from build123d import *

# Parameters (mm, degrees)
ESQUISSE2_R             = 7
BOSS_EXTRU_2_DEPTH      = 22
ENL_V_MAT_EXTRU_1_DEPTH = 19
ESQUISSE5_R             = 5.5
ENL_V_MAT_EXTRU_2_DEPTH = 45
ENL_V_START             = -12
ENL_V_MAT_EXTRU_3_DEPTH = 24


with BuildPart() as part:
    # Esquisse2 → Boss.-Extru.2 (new body, symmetric)
    with BuildSketch(Plane.XY):
        with BuildLine():
            Line((51.296980053, -19), (57, -19))
            Line((57, -19), (86, 15))
            Line((86, 15), (86, 34))
            Line((86, 34), (81, 39))
            Line((81, 39), (57, 39))
            ThreePointArc((57, 39), (48.490791592, 29.99016727), (36.246410316, 28.077357637))
            Line((36.246410316, 28.077357637), (14, 32))
            Line((14, 32), (7, 32))
            Line((7, 32), (0, 25))
            Line((0, 25), (0, 7))
            Line((0, 7), (7, 0))
            Line((7, 0), (39.575538911, 0))
            ThreePointArc((39.575538911, 0), (42.840774692, -1.213413768), (44.521177653, -4.264705882))
            ThreePointArc((44.521177653, -4.264705882), (46.858007856, -12.115672061), (51.296980053, -19))
        make_face()
        with Locations((14, 14)):
            Circle(ESQUISSE2_R, mode=Mode.SUBTRACT)
    extrude(amount=BOSS_EXTRU_2_DEPTH, both=True)

    # Esquisse4 → Enlèv. mat.-Extru.1 (cut)
    with BuildSketch(Plane.XY.offset(22)):
        Polygon((34, 32), (0, 32), (0, -19), (86, -19), (86, 0), (34, 0), align=None)
    extrude(amount=-ENL_V_MAT_EXTRU_1_DEPTH, mode=Mode.SUBTRACT)

    # Esquisse5 → Enlèv. mat.-Extru.2 (cut, through all)
    with BuildSketch(Plane.XY.offset(22)):
        with Locations((72, 25)):
            Circle(ESQUISSE5_R)
    extrude(amount=-ENL_V_MAT_EXTRU_2_DEPTH, mode=Mode.SUBTRACT)

    # Esquisse14 → Enlèv. mat.-Extru.3 (cut)
    with BuildSketch(Plane(origin=(0, 0, -22), x_dir=(-1, 0, 0), z_dir=(0, 0, -1)).offset(ENL_V_START)):
        with BuildLine():
            Line((-75.764705882, 3), (-86, 15))
            Line((-86, 15), (-86, 34))
            Line((-86, 34), (-81, 39))
            Line((-81, 39), (-57, 39))
            ThreePointArc((-57, 39), (-53.002548038, 33.285750119), (-47.224051208, 29.381745985))
            ThreePointArc((-47.224051208, 29.381745985), (-58.169717695, 12.59414375), (-75.764705882, 3))
        make_face()
    extrude(amount=-ENL_V_MAT_EXTRU_3_DEPTH, mode=Mode.SUBTRACT)


solid = part.part
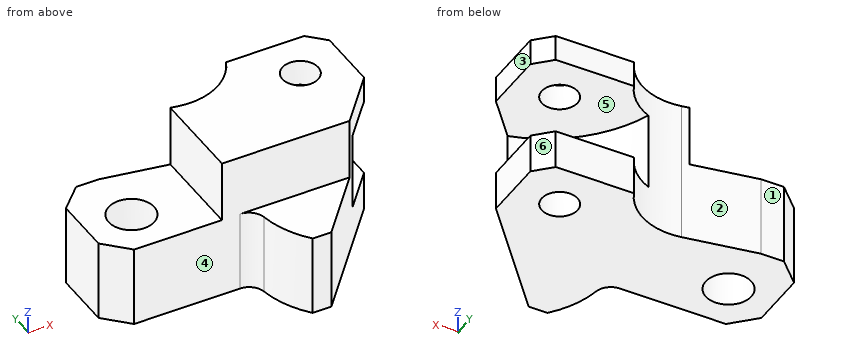
For this review, take the finished solid that the model builds, in its own axes (mm). Face numbers are marked on the shaded views. A direction names the side the tool comes from. Round coordinates to 2 decimals unless told otherwise and drop trailing zeros. Write each loop counter-clockwise with the first axis right and the second up, starting at its lowest first coordinate (ties: lowest second). Pieces come first, ordered by that corner, then holes. Notation, with made-up numbers: (67.25, -26.5) -> (75.25, -26.5) arc R11 cw to (75.25, -20.5) -> close; hole circle Ø8 at (25.5, 8). An arc over 180 degrees is marked (long way). Use CSV: the item, a comma, the result in double quotes.
(1) Consider section B-B, the plane y = 14. Give the boundary of the cut face in (x, z).
Computed values:
outline,"(0, -22) -> (7, -22) -> (7, 3) -> (0, 3) -> close; (21, -22) -> (85.15, -22) -> (85.15, -10) -> (56.72, -10) -> (56.72, 14) -> (85.15, 14) -> (85.15, 22) -> (34, 22) -> (34, 3) -> (21, 3) -> close"
(2) For the marked faces 4, 5 and 6, list the 3-axis set-ups (+Z, -Z, +X, -X, +Y, -Y) from which the entire face can be reached by the end or side of a thin tool; tool diameter is ignored.
Computed values:
face 4,"+Z, -X, -Y"
face 5,"+X, +Y"
face 6,"+Z, -Z, +X, +Y"
(3) Clearance check with flat-ended pins moving along their axes: P1, Ø10, axis at y = 11, z = -12.5, coming from the +X side; P2, Ø5, axis at y = 24, z = 2.5, coming from the +X side; P3, Ø10, axis at y = -5.5, z = -0.5, coming from the -X side (3 decimals); P4, Ø9.5, axis at x = 13, y = 21, coming from the +Z side. State where each tip first meets the part, or that it passes through.
Computed values:
P1,"x = 86"
P2,"x = 50.91"
P3,"x = 41.755"
P4,"z = 3"
(4) Draft analysis for pull direction X (two halves, no side actions). For the marked faces 1, 2 and 3, state which applies: +X half, -X half, draft (parallel to the pull), parting line (faces both ways), or undercut.
Computed values:
face 1,"draft"
face 2,"undercut"
face 3,"+X half"
(5) Consider section C-C, the plane z = 13. Give the boundary of the cut face in (x, y).
Computed values:
outline,"(34, 0) -> (73.21, 0) -> (75.76, 3) arc R41 cw to (47.22, 29.38) arc R19.15 cw to (36.25, 28.08) -> (34, 28.47) -> close"
(6) To check wall thickness, follow L1, parallel to Y at x = 72, z = 16.5; L2, parallel to Y at x = 14, z = -4; L3, parallel to Z at x = 66.5, y = 17. State the ranges of each line that lie inside material, in increasing order. Write a range as [from, to].
Computed values:
L1,"[0, 19.5], [30.5, 39]"
L2,"[0, 7], [21, 32]"
L3,"[-22, -10], [14, 22]"
(7) Consider section D-D, the plane x = 60. Give the boundary of the cut face in (y, z), plus the area to 3 significant figures.
Computed values:
outline,"(-15.48, -22) -> (39, -22) -> (39, -10) -> (11, -10) -> (11, 14) -> (39, 14) -> (39, 22) -> (0, 22) -> (0, 3) -> (-15.48, 3) -> close"
area,"1,430 mm²"
(8) Consider section A-A, the plane z = -1. Give the boundary of the cut face in (x, y).
Computed values:
outline,"(0, 7) -> (7, 0) -> (39.58, 0) arc R5 cw to (44.52, -4.26) arc R29 ccw to (51.3, -19) -> (57, -19) -> (75.76, 3) arc R41 cw to (47.22, 29.38) arc R19.15 cw to (36.25, 28.08) -> (14, 32) -> (7, 32) -> (0, 25) -> close; hole circle Ø14 at (14, 14)"
